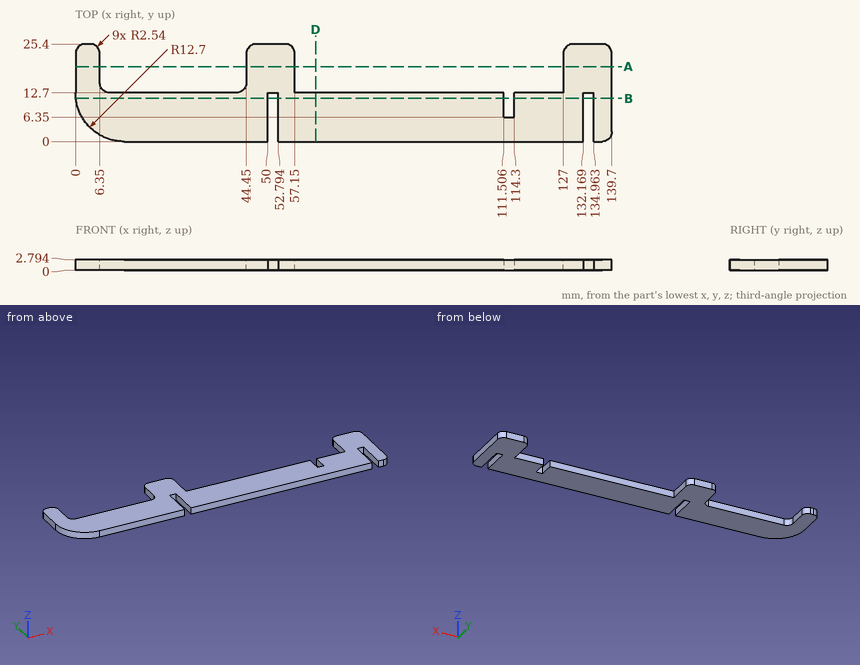
Design review of the part shown in the three views and the two pictorial views. Dimensions are in mm from the part's minimum x, y and z. Coordinates: 2 decimals unless noted, no trailing zeros. Write each loop counter-clockwise with the first axis right and the second up, starting at its lowest first coordinate (ties: lowest second). Pieces come first, ordered by that corner, then holes.
1) We need section B-B on y = 11.25. State the section outline as (x, z) points, then the cut area to 3 significant figures.
2) We need section D-D on x = 62.5. State the section outline as (y, z) points.
3) We need section A-A on y = 19.5. State the section outline as (x, z) points, then the cut area to 3 significant figures.
4) To check wall thickness, follow probe 1 along X at (y, z) = (19.5, 0.65); probe 2 along X at (y, z) = (24.25, 0.95); probe 3 along X at (y, z) = (8.5, 0.35) (1 decimal). State the ranges of each line that lie inside material, in increasing order.
5) Clearance check with flat-ended pins moving along their axes: pin 1 Ø1.4 at (y, z) = (9, 2) entering from -X; pin 2 Ø1.4 at (x, z) = (93, 1.5) entering from +Y; pin 3 Ø1.4 at (y, z) = (8, 1) entering from -X. State where each tip first meets the part, or that it passes through.
Answer list:
1. outline: (0.08, 0) - (50, 0) - (50, 2.79) - (0.08, 2.79) - close; (52.79, 0) - (111.51, 0) - (111.51, 2.79) - (52.79, 2.79) - close; (114.3, 0) - (132.17, 0) - (132.17, 2.79) - (114.3, 2.79) - close; (134.96, 0) - (139.7, 0) - (139.7, 2.79) - (134.96, 2.79) - close
1. area: 367 mm2
2. outline: (0, 0) - (12.7, 0) - (12.7, 2.79) - (0, 2.79) - close
3. outline: (0, 0) - (6.35, 0) - (6.35, 2.79) - (0, 2.79) - close; (44.45, 0) - (57.15, 0) - (57.15, 2.79) - (44.45, 2.79) - close; (127, 0) - (139.7, 0) - (139.7, 2.79) - (127, 2.79) - close
3. area: 88.7 mm2
4. probe 1: x = 0 to 6.35, 44.45 to 57.15, 127 to 139.7
4. probe 2: x = 0.41 to 5.94, 44.86 to 56.74, 127.41 to 139.29
4. probe 3: x = 0.7 to 50, 52.8 to 111.5, 114.3 to 132.2, 135 to 139.7
5. pin 1: stops at x = 0.36
5. pin 2: stops at y = 12.7
5. pin 3: stops at x = 0.65
